Could you check a few things on this model? Use its own coordinates, in mm. A direction names the side the tool comes from. Give positions to 0.01 mm unless a question says otherwise; leave off trailing zeros. Order: outer loops, then holes, each group sorted by start corner. A loop starts at its lowest first (then second) coordinate and runs counter-clockwise, first axis right, second up. Notation, with made-up numbers: (68.25, 20.5) -> (81.25, 20.5) arc R18 ccw to (81.25, 50.5) -> close; hole circle Ø4 at (30.5, -35.5). An arc over 180 degrees is marked (long way). Answer as CSV lines item,"result". Start each with the question number.
(1) We'd pull the mould along X, two halves only. Please class faces 3 (the face through (0, 12.7, -4)), 4 (the face through (12.7, 0, -4)), 5 (the face through (-12.7, 0, -4)), 6 (the face through (0, -9.525, -4)): released by +X, released by -X, zero draft, split by the parting line, or undercut.
(2) On a 3-axis mill with a long thin cutter (end or side, diameter ignored), from which of +Z, -Z, +X, -X, +Y, -Y can I reach the whole of each face in a straight line? I mean faces 1 (the face through (11, 0, 285.75)), 2 (the face through (-9.525, 0, -4)). Say none if no direction works.
(3) I want a section at A-A (z = 226). Please give me the cut outline in (x, y) (3 decimals).
(4) I want a section at B-B (x = -1). Please give me the cut outline in (y, z) (3 decimals).
(5) Will this pin go through, and if not, where does the flat tip stop? pin 1 Ø8 at (x, y) = (-7, -8) entering from -Z.
(6) I need wall thicknesses on L1, parallel to Y at x = -8.5, z = -148.5 (3 decimals). Which ranges of the line are inside material? Lowest first, please.
Autodesk Inventor part; units mm, degrees
ref_plane "YZ Plane" through (0, 0, 0) normal (1, 0, 0) x (0, 1, 0)
ref_plane "XZ Plane" through (0, 0, 0) normal (0, 1, 0) x (-1, 0, 0)
ref_plane "XY Plane" through (0, 0, 0) normal (0, 0, 1) x (1, 0, 0)
sketch "Sketch1" plane through (0, 0, 0) normal (0, 0, 1) x (1, 0, 0)
  line L0 (-17.78, 0) -> (17.78, 0)
  line L1 (0, -17.78) -> (0, 17.78)
  line L2 (-12.7, 12.7) -> (12.7, 12.7)
  line L3 (12.7, 12.7) -> (12.7, -12.7)
  line L4 (12.7, -12.7) -> (-12.7, -12.7)
  line L5 (-12.7, -12.7) -> (-12.7, 12.7)
  line L6 (9.525, 9.525) -> (-9.525, 9.525)
  line L7 (-9.525, 9.525) -> (-9.525, -9.525)
  line L8 (-9.525, -9.525) -> (9.525, -9.525)
  line L9 (9.525, -9.525) -> (9.525, 9.525)
  point P0 (0, 0)
  point P1 (-12.7, 0)
  point P2 (0, 12.7)
  dimension "d0" = 25.4
  dimension "d1" = 3.175
extrude "Extrusion1" add sketch "Sketch1" along normal mid plane 571.5 contours L5 L2 L1 L6 L7 L0 | L0 L7 L8 L1 L4 L5 | L1 L8 L9 L0 L3 L4 | L2 L3 L0 L9 L6 L1
properties part number "tubing_template_0.125" material "Aluminum-6061"
Final values:
1,face 3,"zero draft"
1,face 4,"released by +X"
1,face 5,"released by -X"
1,face 6,"undercut"
2,face 1,"+Z, +X, -X, +Y, -Y"
2,face 2,"+Z, -Z"
3,outline,"(-12.7, -12.7) -> (12.7, -12.7) -> (12.7, 12.7) -> (-12.7, 12.7) -> close; hole (-9.525, -9.525) -> (9.525, -9.525) -> (9.525, 9.525) -> (-9.525, 9.525) -> close"
4,outline,"(-12.7, -285.75) -> (-9.525, -285.75) -> (-9.525, 285.75) -> (-12.7, 285.75) -> close; (9.525, -285.75) -> (12.7, -285.75) -> (12.7, 285.75) -> (9.525, 285.75) -> close"
5,pin 1,"z = -285.75"
6,L1,"-12.7 to -9.525, 9.525 to 12.7"
